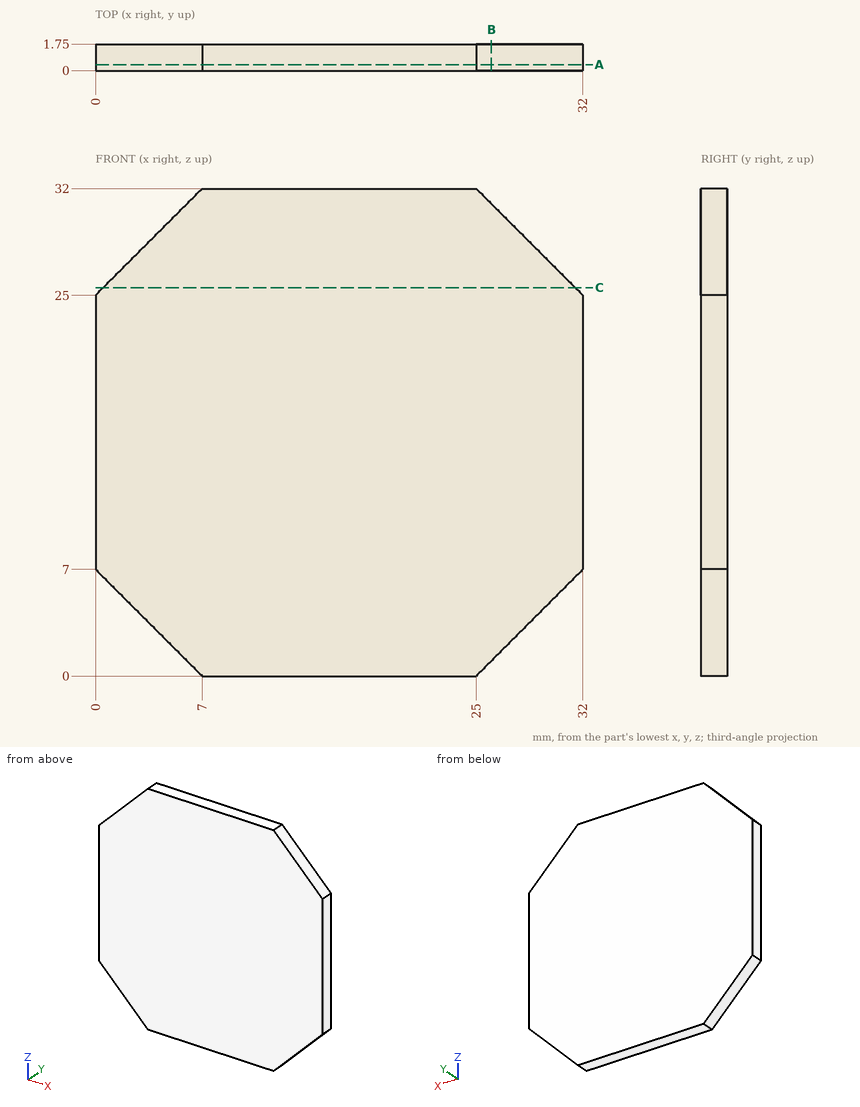
Check sheet for the drawn part. Datum: minimum x, y, z corner. Units: mm. Give positions to 0.01 mm unless a question says otherwise; leave off trailing zeros. Write each loop counter-clockwise with the first axis right and the second up, starting at its lowest first coordinate (ties: lowest second). Pieces come first, ordered by that corner, then holes. Notation, with made-up numbers: M 34.5,35.5 L 75.5,35.5 A23 ccw 75.5,44.5 Z; hole C 40,-4 d8. An arc over 180 degrees is marked long. Write item = value, one per line.
(1) Material ranges on line 1 (Z direction, x = 29, y = 0.6); line 2 (X direction, y = 0.95, z = 27); line 3 (Z direction, x = 6, y = 1.45), recorded low to high.
Found:
line_1 = 4 to 28
line_2 = 2 to 30
line_3 = 1 to 31
(2) Sectioned sample at C-C (z = 25.5). Record the cut outline in (x, y).
Found:
outline = M 0.5,0 L 31.5,0 L 31.5,1.75 L 0.5,1.75 Z
(3) Sectioned sample at B-B (x = 26). Record the cut outline in (y, z), then the cut area to 3 significant figures.
Found:
outline = M 0,1 L 1.75,1 L 1.75,31 L 0,31 Z
area = 52.5 mm2
(4) Sectioned sample at A-A (y = 0.4). Record the cut outline in (x, z).
Found:
outline = M 0,7 L 7,0 L 25,0 L 32,7 L 32,25 L 25,32 L 7,32 L 0,25 Z
